Geometry check sheet. Reference: the model listing, model coordinates, mm. Give positions to 0.01 mm unless a question says otherwise; leave off trailing zeros. Write each loop counter-clockwise with the first axis right and the second up, starting at its lowest first coordinate (ties: lowest second). Pieces come first, ordered by that corner, then holes.
(1) Cross-section at A-A (y = 4.15). Count the separate pieces of the cut face and the enclosed holes in it, and give its area (3 significant figures).
(2) Cross-section at C-C (x = -155). Record the boundary of the cut face in (y, z), and give its area (3 significant figures).
(3) Thickness scan on line 1 along X through (y, z) = (3.3, 32); line 2 along X through (y, z) = (3.4, 28.5); line 3 along Z through (x, y) = (-222.5, 1.25). Record the ranges inside material, lowest first.
(4) Depth check by flat-ended pin: P1, Ø3.5, axis at x = 0, z = -300, coming from the -Y side; P2, Ø1, axis at y = 4, z = -193, coming from the -X side; P3, Ø1.5, axis at x = 238, y = 3, coming from the +Z side. Enter the tip coordinate at first touch or a pass-through.
(5) Cross-section at B-B (z = 123.5). Record the boundary of the cut face in (x, y).
Autodesk Inventor part; units mm, degrees
ref_plane "YZ Plane" through (0, 0, 0) normal (1, 0, 0) x (0, 1, 0)
ref_plane "XZ Plane" through (0, 0, 0) normal (0, 1, 0) x (-1, 0, 0)
ref_plane "XY Plane" through (0, 0, 0) normal (0, 0, 1) x (1, 0, 0)
sketch "Sketch1" plane through (0, 0, 0) normal (0, 1, 0) x (-1, 0, 0)
  line L0 (-500, 500) -> (500, 500)
  line L1 (500, 500) -> (500, -500)
  line L2 (500, -500) -> (-500, -500)
  line L3 (-500, -500) -> (-500, 500)
  line L4 (-500, 500) -> (500, -500) construction
  line L5 (500, 500) -> (-500, -500) construction
  point P0 (0, 0)
  dimension "d0" = 1000
  dimension "d1" = 1000
extrude "Extrusion1" add sketch "Sketch1" along normal blind 6
sketch "Sketch2" plane through (0, 0, 0) normal (0, -1, 0) x (1, 0, 0)
  circle A0 centre (0, 0) radius 310
  dimension "d4" = 620
extrude "Extrusion2" cut sketch "Sketch2" against normal blind 10 keep common part
sketch "Sketch3" plane through (0, 0, 0) normal (0, -1, 0) x (1, 0, 0)
  circle A0 centre (0, 0) radius 300 construction
  line L0 (0, -434) -> (0, 434) construction
  point P0 (0, 300)
  dimension "d7" = 600
hole "Hole1" at (0, 0, 300) direction (0, 1, 0) diameter 6 end through all
pattern_circular "Circular Pattern1" count 8 over 360 about axis through (0, 0, 0) along (0, 1, 0) of "Hole1"
properties part number "płyta 6 biala okragla R600"
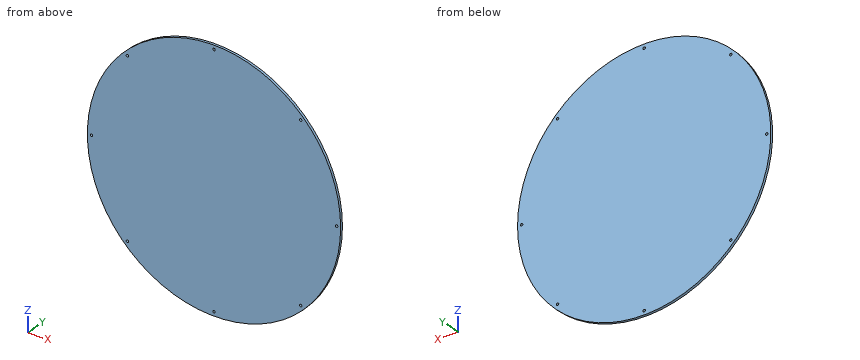
Reply:
1. separate pieces: 1
1. enclosed holes: 8
1. area: 302,000 mm2
2. outline: (0, -268.47) - (6, -268.47) - (6, 268.47) - (0, 268.47) - close
2. area: 3,220 mm2
3. line 1: x = -308.34 to 308.34
3. line 2: x = -308.69 to 308.69
3. line 3: z = -215.86 to 215.86
4. P1: passes through
4. P2: stops at x = -242.99
4. P3: stops at z = 199.53
5. outline: (-284.34, 0) - (284.34, 0) - (284.34, 6) - (-284.34, 6) - close
